Autodesk Inventor part; units mm, degrees
ref_plane "YZ Plane" through (0, 0, 0) normal (1, 0, 0) x (0, 1, 0)
ref_plane "XZ Plane" through (0, 0, 0) normal (0, 1, 0) x (-1, 0, 0)
ref_plane "XY Plane" through (0, 0, 0) normal (0, 0, 1) x (1, 0, 0)
sketch "Эскиз1" plane through (0, 0, 0) normal (0, 0, 1) x (1, 0, 0)
  line L0 (0, 0) -> (20, 0)
  line L1 (20, 0) -> (20, 25)
  line L2 (16, 29) -> (4, 29)
  line L3 (0, 25) -> (0, 0)
  line L4 (4, 29) -> (0, 25)
  line L5 (16, 29) -> (20, 25)
  point P0 (20, 29)
  point P1 (0, 29)
  dimension "d12" = 20
  dimension "d13" = 29
  dimension "d14" = 4
  dimension "d15" = 4
  dimension "d16" = 4
  dimension "d17" = 4
revolve "Вращение2" add sketch "Эскиз1" angle 360 about axis through (0, 0, 0) along (1, 0, 0)
sketch "Эскиз4" plane through (0, 0, 0) normal (0, 0, 1) x (1, 0, 0)
  line L0 (0, -25) -> (0, 25) construction
  line L1 (0, 4) -> (9, 4)
  line L2 (9, 4) -> (9, -4)
  line L3 (9, -4) -> (0, -4)
  line L4 (0, -4) -> (0, 4)
  point P0 (0, 0)
  point P1 (0, 0)
  point P2 (0, 0)
  dimension "d23" = 9
  dimension "d24" = 8
extrude "Выдавливание3" cut sketch "Эскиз4" along normal through all both and the other way through all
properties part number "711113"
CAD build for the part. Positions are in the model's coordinates, mm. A direction names the side the tool comes from. Coordinates: 2 decimals unless noted, no trailing zeros. Write each loop counter-clockwise with the first axis right and the second up, starting at its lowest first coordinate (ties: lowest second). Pieces come first, ordered by that corner, then holes. Notation, with made-up numbers: M 60.5,38.5 L 81.5,38.5 A31 cw 81.5,69.5 Z; hole C 72.5,31.25 d5. An arc over 180 degrees is marked long. Answer as a JSON object with one key per item and string values. Group by question number.
1) Pin check, flat tips, straight feed: pin 1 Ø10 at (x, y) = (2.5, 4.5) entering from -Z; pin 2 Ø10 at (x, z) = (5, 12.5) entering from +Y; pin 3 Ø5 at (y, z) = (-19.5, -20.5) entering from -X. Stop position of each tip, or through.
2) Tool access for faces 4 (the face through (9, 0, 0)), 5 (the face through (0, 12, 0)): list every direction of +Z, -Z, +X, -X, +Y, -Y with a clear straight run to the whole face (end or side of a thin tool).
3) Saw through at D-D (x = 11.5). Write the cut outline in (y, z), plus the area to 3 significant figures.
4) Mould opens along Y. For faces 1 (the face through (0, -12, 0)), 2 (the face through (0.25, -25.245, 0.506)), 3 (the face through (4, 4, 0)) say: +Y half, -Y half, draft (parallel to the pull), parting line (faces both ways), or undercut.
5) Saw through at B-B (x = 7.25). Write the cut outline in (y, z), plus the area to 3 significant figures.
6) Wall check: line 1 (Y direction, x = 4, z = 1.5); line 2 (X direction, y = -1.5, z = 12.5); line 3 (Y direction, x = 3.75, z = 2). Give the ranges that are in metal, low to high. Write a range as from..to.
7) Saw through at A-A (z = 0). Write the cut outline in (x, y), plus the area to 3 significant figures.
8) Saw through at C-C (y = 0). Write the cut outline in (x, z).
Values follow:
{
 "1": {"pin 1": "stops at z = -28.72", "pin 2": "stops at y = 28.01", "pin 3": "stops at x = 0.79"},
 "2": {"face 4": "+Z, -Z, -X", "face 5": "+Z, -Z, -X, +Y, -Y"},
 "3": {"outline": "C 0,0 d58", "area": "2,640 mm2"},
 "4": {"face 1": "draft", "face 2": "-Y half", "face 3": "undercut"},
 "5": {"outline": "M -4,-28.72 L -4,28.72 A29 ccw Z; M 4,-28.72 A29 ccw 4,28.72 Z", "area": "2,180 mm2"},
 "6": {"line 1": "y = -28.96..-4, 4..28.96", "line 2": "x = 9..20", "line 3": "y = -28.68..-4, 4..28.68"},
 "7": {"outline": "M 0,-25 L 4,-29 L 16,-29 L 20,-25 L 20,25 L 16,29 L 4,29 L 0,25 L 0,4 L 9,4 L 9,-4 L 0,-4 Z", "area": "1,060 mm2"},
 "8": {"outline": "M 9,-29 L 16,-29 L 20,-25 L 20,25 L 16,29 L 9,29 Z"}
}
